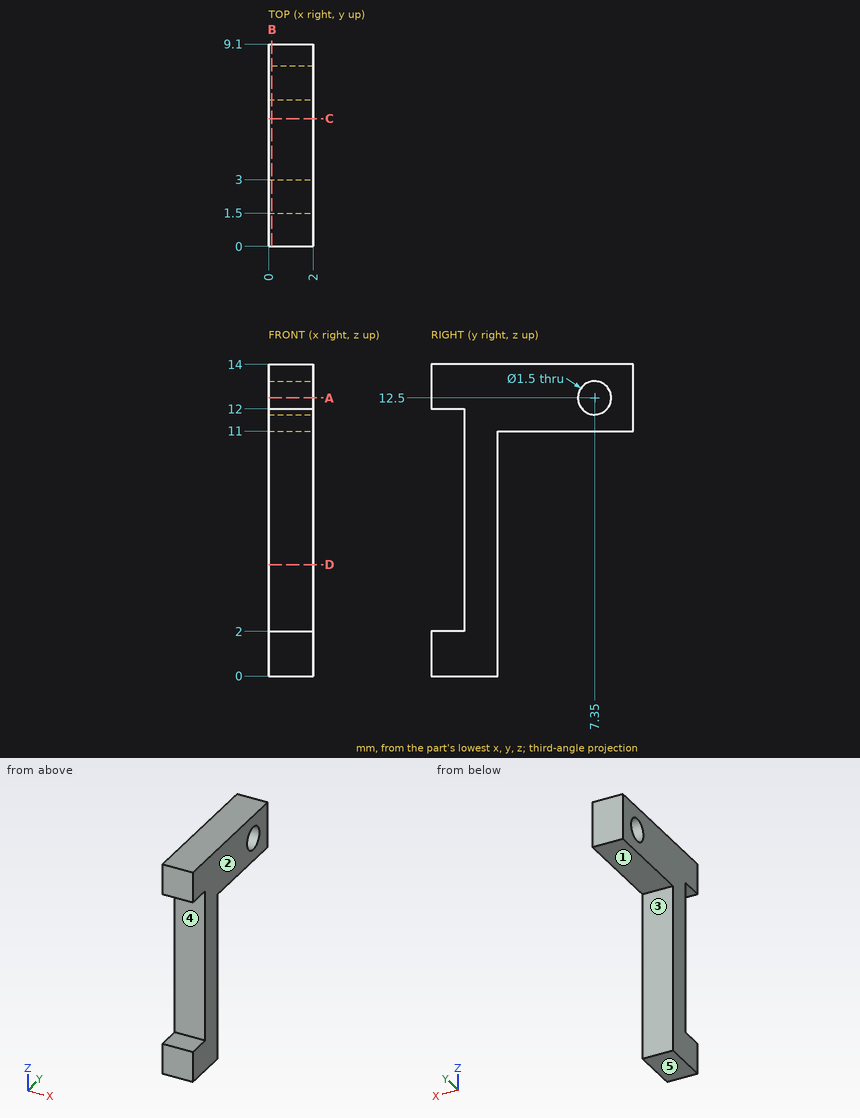
Geometry check sheet. Reference: drawing and pictorial views, mm from the part's lowest x, y, z. A direction names the side the tool comes from. Coordinates: 2 decimals unless noted, no trailing zeros. Write each loop counter-clockwise with the first axis right and the second up, starting at its lowest first coordinate (ties: lowest second). Pieces come first, ordered by that corner, then holes. Notation, with made-up numbers: (-2, 51.5) - (47, 51.5) arc R23 ccw to (47, 75.5) - close; hole circle Ø10 at (10, -6.75). An arc over 180 degrees is marked (long way). One line per question, with ' | ' between items. Start each with the question number.
1. Section check B-B (x = 0.15). Enter the section's corners in (y, z), plus the area to 3 significant figures.
2. Draft check along Z on the marked faces 3, 4 and 5. Enter one of: released by +Z, released by -Z, zero draft, split by the parting line, or undercut.
3. Section check D-D (z = 5). Enter the section's corners in (x, y).
4. Material ranges on line 1 along Z through (x, y) = (0.4, 4.5); line 2 along Z through (x, y) = (1.4, 1.25); line 3 along Z through (x, y) = (0.25, 7.5), recorded low to high.
5. Section check A-A (z = 12.5). Enter the section's corners in (x, y).
6. Gauge pin test, flat ends, axial feed: P1, Ø0.6, axis at x = 1, z = 9, coming from the -Y side; P2, Ø1, axis at x = 1.5, z = 10, coming from the +Y side; P3, Ø0.9, axis at y = 7.35, z = 12.5, coming from the -X side. Record the tip position at first contact, or that the pin passes through.
7. Section check C-C (y = 5.75). Enter the section's corners in (x, z).
8. Access from +Z, -Z, +X, -X, +Y, -Y to the whole of each face (thin tool, end or side, straight path). Record for the marked faces 1 and 2.
Computed values:
1) outline: (0, 0) - (3, 0) - (3, 11) - (9.1, 11) - (9.1, 14) - (0, 14) - (0, 12) - (1.5, 12) - (1.5, 2) - (0, 2) - close; hole circle Ø1.5 at (7.35, 12.5) | area: 43.5 mm²
2) face 3: zero draft | face 4: undercut | face 5: released by -Z
3) outline: (0, 1.5) - (2, 1.5) - (2, 3) - (0, 3) - close
4) line 1: 11 to 14 | line 2: 0 to 2, 12 to 14 | line 3: 11 to 11.77, 13.23 to 14
5) outline: (0, 0) - (2, 0) - (2, 6.6) - (0, 6.6) - close; (0, 8.1) - (2, 8.1) - (2, 9.1) - (0, 9.1) - close
6) P1: y = 1.5 | P2: y = 3 | P3: through
7) outline: (0, 11) - (2, 11) - (2, 14) - (0, 14) - close
8) face 1: -Z, +X, -X, +Y | face 2: +Z, -Z, +X, +Y, -Y
